Read the model definition and answer for the solid it produces. Units are mm, in the model's axes. Face numbers are marked on the shaded views. A direction names the side the tool comes from. Coordinates: 2 decimals unless noted, no trailing zeros. Write each loop counter-clockwise with the first axis right and the second up, starting at its lowest first coordinate (ties: lowest second). Pieces come first, ordered by that corner, then holes.
(1) Section C-C on x = 4.4 is taken. Write down the section's boundary in (y, z).
(2) Given pin 1 (0.7 mm diameter, centred on y = 0.5, z = -0.5, fed in from -X), flat-ended and moving along its own axis, determine where the tip first touches the part or whether it passes through.
(3) The mould has two halves that part along Y. Classify the marked faces 1, 2 and 3: +Y half, -Y half, draft (parallel to the pull), parting line (faces both ways), or undercut.
(4) Section A-A on x = 0.7 is taken. Write down the section's boundary in (y, z).
(5) Find the intervals of material crossed by probe 1 along Y at (x, z) = (3.1, 0.95); probe 2 along Z at (x, y) = (0.75, -0.2); probe 3 along Z at (x, y) = (1.45, -0.8), in increasing order.
(6) Which of the six approach directions +Z, -Z, +X, -X, +Y, -Y give full straight-line access (tool end or side, diameter ignored) to the marked faces 4, 5 and 6?
(7) Section B-B on x = 2.4 is taken. Write down the section's boundary in (y, z).
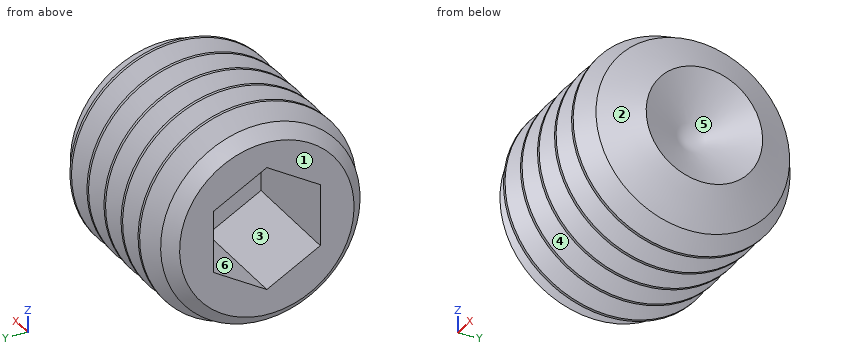
from build123d import *

# Parameters (mm, degrees)
CUT_EXTRUDE1_DEPTH = 2.54


with BuildPart() as part:
    # Sketch1 → Revolve1 (revolve)
    with BuildSketch(Plane(origin=(0, 0, 0), x_dir=(-1, 0, 0), z_dir=(0, 0, -1)), mode=Mode.PRIVATE) as revolve1_sk:
        Polygon((-4.7625, 1.2954), (-3.984145154, 0), (0, 0), (0, 1.94056), (-0.277871959, 2.218431959), (-0.47244, 1.94056), (-0.803246049, 2.413), (-0.870596619, 2.413), (-1.201402668, 1.94056), (-1.532208718, 2.413), (-1.599559287, 2.413), (-1.930365336, 1.94056), (-2.261171385, 2.413), (-2.328521955, 2.413), (-2.659328004, 1.94056), (-2.990134054, 2.413), (-3.057484623, 2.413), (-3.388290672, 1.94056), (-3.719096722, 2.413), (-3.786447291, 2.413), (-4.11725334, 1.94056), (-4.266750263, 2.154063732), align=None)
    revolve(revolve1_sk.sketch.rotate(Axis((4.762525, 0, 0), (-1, 0, 0)), 270), axis=Axis((4.762525, 0, 0), (-1, 0, 0)))

    # Sketch2 → Cut-Extrude1 (cut)
    with BuildSketch(Plane.ZY):
        Polygon((1.374082094, 0), (0.687041047, 1.18999), (-0.687041047, 1.18999), (-1.374082094, 0), (-0.687041047, -1.18999), (0.687041047, -1.18999), align=None)
    extrude(amount=-CUT_EXTRUDE1_DEPTH, mode=Mode.SUBTRACT)


solid = part.part
Response:
1. outline: circle Ø3.85 at (0, 0); hole circle Ø1.38 at (0, 0)
2. pin 1: stops at x = 2.54
3. face 1: draft
3. face 2: parting line
3. face 3: undercut
4. outline: circle Ø4.53 at (0, 0); hole (-1.19, -0.69) - (0, -1.37) - (1.19, -0.69) - (1.19, 0.69) - (0, 1.37) - (-1.19, 0.69) - close
5. probe 1: y = -2.15 to 2.15
5. probe 2: z = -2.33 to -1.26, 1.26 to 2.33
5. probe 3: z = -2.15 to -0.91, 0.91 to 2.15
6. face 4: none
6. face 5: +X
6. face 6: -X
7. outline: circle Ø4.62 at (0, 0); hole (-1.19, -0.69) - (0, -1.37) - (1.19, -0.69) - (1.19, 0.69) - (0, 1.37) - (-1.19, 0.69) - close
